The figure shows three views and two pictorial views of one solid part (mm, origin at its lowest corner). Answer the questions. A direction names the side the tool comes from. Give positions to 0.01 mm unless a question says otherwise; leave off trailing zeros. Write each loop counter-clockwise with the first axis right and the second up, starting at its lowest first coordinate (ties: lowest second). Pieces come first, ordered by that corner, then holes. Notation, with made-up numbers: M 81,5.5 L 101,5.5 A19 cw 101,19.5 Z; hole C -4,-29 d11. An arc over 180 degrees is marked long. Return JSON: item names as keys, results as strings.
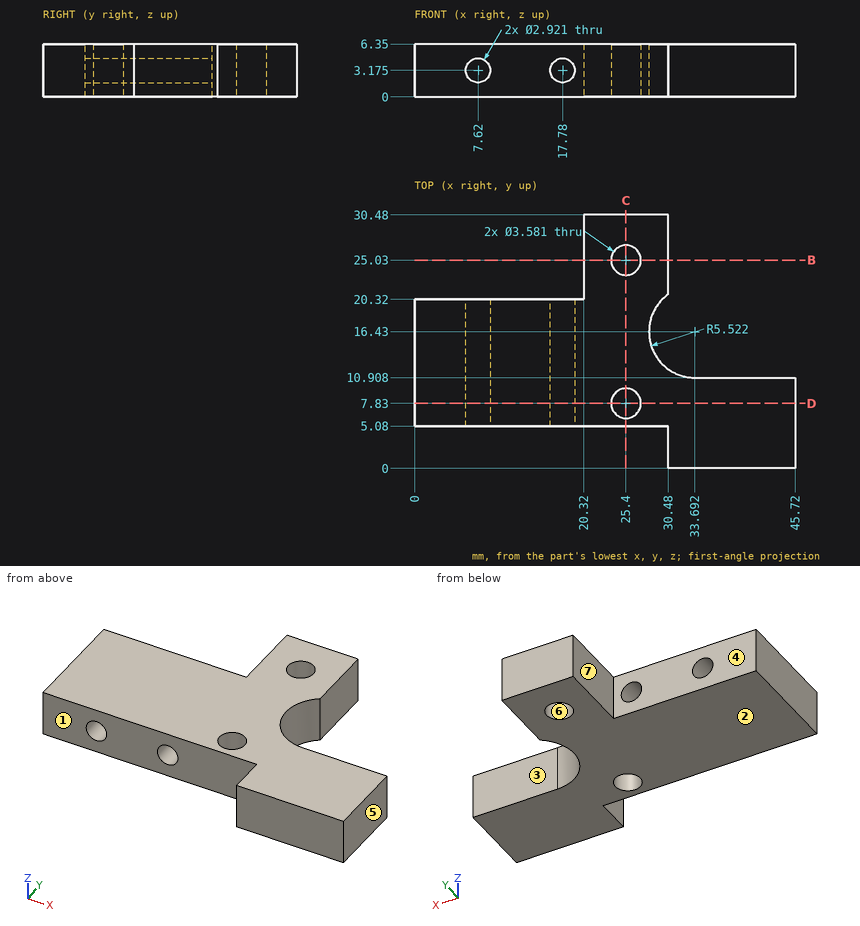
Item 1: Given pin 1 Ø1.5 at (y, z) = (26, 4.5) entering from -X; pin 2 Ø2.5 at (y, z) = (3, 3.5) entering from -X; pin 3 Ø3 at (x, y) = (25.4, 25.03) entering from +Z; pin 4 Ø3 at (x, z) = (8, 2.5) entering from -Y, each flat-ended and moving along its own axis, determine where each tip first touches the part or whether it passes through.
Geometry results:
{"pin 1": "stops at x = 20.32", "pin 2": "stops at x = 30.48", "pin 3": "passes through", "pin 4": "stops at y = 5.08"}
Item 2: A cutting plane is placed at B-B, the plane y = 25.03. Write down the section's boundary in (x, z).
Geometry results:
{"outline": "M 20.32,0 L 23.61,0 L 23.61,6.35 L 20.32,6.35 Z; M 27.19,0 L 30.48,0 L 30.48,6.35 L 27.19,6.35 Z"}
Item 3: A cutting plane is placed at C-C, the plane x = 25.4. Write down the section's boundary in (y, z).
Geometry results:
{"outline": "M 5.08,0 L 6.04,0 L 6.04,6.35 L 5.08,6.35 Z; M 9.62,0 L 23.24,0 L 23.24,6.35 L 9.62,6.35 Z; M 26.82,0 L 30.48,0 L 30.48,6.35 L 26.82,6.35 Z"}
Item 4: Which of the six approach directions +Z, -Z, +X, -X, +Y, -Y give full straight-line access (tool end or side, diameter ignored) to the marked faces 1, 2, 3 and 4?
Geometry results:
{"face 1": "+Z, -Z, -X, -Y", "face 2": "-Z, +X, -X, +Y, -Y", "face 3": "+Z, -Z, +X, +Y", "face 4": "+Z, -Z, -X, +Y"}
Item 5: Determine the mould class of the marked faces 5, 6 and 7 for opening direction X: +X half, -X half, draft (parallel to the pull), parting line (faces both ways), or undercut.
Geometry results:
{"face 5": "+X half", "face 6": "undercut", "face 7": "-X half"}
Item 6: Find the intervals of material crossed by line 1 (Y direction, x = 25.4, z = 4.25); line 2 (X direction, y = 10, z = 4.5) (1 decimal); line 3 (Y direction, x = 22, z = 3.5), in increasing order.
Geometry results:
{"line 1": "y = 5.08 to 6.04, 9.62 to 23.24, 26.82 to 30.48", "line 2": "x = 0 to 7, 8.2 to 17.2, 18.4 to 45.7", "line 3": "y = 5.08 to 30.48"}
Item 7: A cutting plane is placed at D-D, the plane y = 7.83. Count the separate pieces of the cut face and the enclosed holes in it, plus the area to 3 significant figures.
Geometry results:
{"separate pieces": "2", "enclosed holes": "2", "area": "254 mm2"}
